Build history of the part. All positions in model axes, mm. A direction names the side the tool comes from. Round coordinates to 2 decimals unless told otherwise and drop trailing zeros. Loops run counter-clockwise (first coordinate to the right, second up) from the corner with the lowest first, then second, coordinate; pieces in that order, holes last. Notation, with made-up numbers: (10, 34.25) - (43, 34.25) arc R19 cw to (43, 38.25) - close; hole circle Ø10 at (20.5, -32.75). An arc over 180 degrees is marked (long way). Use a Markdown table: item, result.
from build123d import *

# Parameters (mm, degrees)
SKETCH_1_W                  = 16
SKETCH_1_H                  = 120
EXTRUDE_1_DEPTH             = 10
CHAMFER_1_SIZE              = 1
HOLE_WIZARD_M61_D           = 6.6
HOLE_WIZARD_M61_CBORE_D     = 11
HOLE_WIZARD_M61_CBORE_DEPTH = 6


with BuildPart() as part:
    # Эскиз1 → Бобышка-Вытянуть1 (new body)
    with BuildSketch(Plane(origin=(0, 0, 0), x_dir=(1, 0, 0), z_dir=(0, 1, 0))):
        Rectangle(SKETCH_1_W, SKETCH_1_H)
    extrude(amount=-EXTRUDE_1_DEPTH)

    # Фаска1
    chamfer_1_edges = [part.edges().sort_by_distance(p)[0] for p in [
        (0, 0, 60),
        (-8, 0, 0),
        (0, 0, -60),
        (8, 0, 0),
    ]]
    chamfer(chamfer_1_edges, length=CHAMFER_1_SIZE)

    # Цековка для винта с внутренним шестигранником M61 (through all)
    with Locations(Plane(origin=(0, 0, 0), x_dir=(-1, 0, 0), z_dir=(0, 1, 0))):
        with Locations((0, 30), (0, -30)):
            CounterBoreHole(HOLE_WIZARD_M61_D / 2, HOLE_WIZARD_M61_CBORE_D / 2, HOLE_WIZARD_M61_CBORE_DEPTH)


solid = part.part
Q1. Pull direction Z, two halves, no side cores. Call faces 1 (the face through (0, -5, -60)), 2 (the face through (0, -10, -1)), 3 (the face through (0.716, -2.958, 35.453)): pulls with the +Z half, pulls with the -Z half, needs draft (parallel to the pull), parting line crosses it, or undercut.
Results found:
| item | result |
|---|---|
| face 1 | pulls with the -Z half |
| face 2 | needs draft |
| face 3 | undercut |
Q2. Cut at B-B, the plane x = 0. List the corners of the cut face in (y, z), plus the area to 3 significant figures.
Results found:
| item | result |
|---|---|
| outline | (-10, -60) - (-1, -60) - (0, -59) - (0, -35.5) - (-6, -35.5) - (-6, -33.3) - (-10, -33.3) - close; (-10, -26.7) - (-6, -26.7) - (-6, -24.5) - (0, -24.5) - (0, 24.5) - (-6, 24.5) - (-6, 26.7) - (-10, 26.7) - close; (-10, 33.3) - (-6, 33.3) - (-6, 35.5) - (0, 35.5) - (0, 59) - (-1, 60) - (-10, 60) - close |
| area | 1,010 mm2 |
Q3. Cut at A-A, the plane z = -30. List the corners of the cut face in (x, y), plus the area to 3 significant figures.
Results found:
| item | result |
|---|---|
| outline | (-8, -10) - (-3.3, -10) - (-3.3, -6) - (-5.5, -6) - (-5.5, 0) - (-7, 0) - (-8, -1) - close; (3.3, -10) - (8, -10) - (8, -1) - (7, 0) - (5.5, 0) - (5.5, -6) - (3.3, -6) - close |
| area | 66.6 mm2 |
Q4. Cut at C-C, the plane y = -7.75. List the corners of the cut face in (x, z).
Results found:
| item | result |
|---|---|
| outline | (-8, -60) - (8, -60) - (8, 60) - (-8, 60) - close; hole circle Ø6.6 at (0, -30); hole circle Ø6.6 at (0, 30) |
Q5. Which spindle directions (+Z, -Z, +X, -X, +Y, -Y) get a long thin tool onto all of the face, cutting with end or side? Do faces 4 (the face through (-4, -6, -30)), 5 (the face through (0, -5, 60)). Say none if no direction does.
Results found:
| item | result |
|---|---|
| face 4 | +Y |
| face 5 | +Z, +X, -X, +Y, -Y |
Q6. Probe line 1 (Z direction, x = 3, y = -7.5); line 2 (Z direction, x = 2, y = -9); line 3 (X direction, y = -1.5, z = -25). List the from-to ranges inside material, lowest first.
Results found:
| item | result |
|---|---|
| line 1 | z = -60 to -31.37, -28.63 to 28.63, 31.37 to 60 |
| line 2 | z = -60 to -32.62, -27.38 to 27.38, 32.62 to 60 |
| line 3 | x = -8 to -2.29, 2.29 to 8 |
Q7. Drop a flat-ended pin along its axis: pin 1 (5.5 mm diameter, centred on x = -0.5, z = 32, fed in from +Y). Give the stop position or say it passes through.
Results found:
| item | result |
|---|---|
| pin 1 | stops at y = -6 |
